Verification items for the finished model (mm, model axes). Round coordinates to 2 decimals unless told otherwise and drop trailing zeros. Order: outer loops, then holes, each group sorted by start corner. A loop starts at its lowest first (then second) coordinate and runs counter-clockwise, first axis right, second up. Notation, with made-up numbers: M 19,86.25 L 64,86.25 A28 ccw 64,122.25 Z; hole C 49,-30.5 d7. An arc over 180 degrees is marked long. Use one line per item in the form item = value. Start each with the question number.
Item 1: Thickness scan on probe 1 along Y at (x, z) = (-1.05, 21.75); probe 2 along X at (y, z) = (-1469, 3.25); probe 3 along Y at (x, z) = (1.15, 18.5). Record the ranges inside material, lowest first. Write a range as [from, to].
Item 2: Cross-section at B-B on y = -1652. Enter the section's corners in (x, z).
Item 3: Cross-section at A-A on z = 8.5. Enter the section's corners in (x, y), then the cut area to 3 significant figures.
Item 4: Go/stop test with a flat-tipped pin: pin 1 Ø2 at (x, y) = (-10, -1359.5) entering from -Z. Record where the tip stops, or that it passes through.
from build123d import *

# Parameters (mm, degrees)
F0_W     = 3.9
F0_H     = 3
F0_W_2   = 4.1
F0_H_2   = 5.1741511822
F1_DEPTH = 2000
F3_D     = 2
F4_W     = 32.8
F4_H     = 100
F5_DEPTH = 25.0010018114


with BuildPart() as f1:
    # F0 (on Front) → F1 (new body)
    with BuildSketch(Plane.XZ):
        with Locations((14.5, 1.7925839761)):
            Rectangle(F0_W, F0_H)
        Polygon((-16.35, 25.2925857875), (-16.35, 0.2925839761), (-12.45, 0.2925839761), (-12.45, 3.2925839761), (-12.45, 8.4667351583), (-8.35, 8.4667351583), (-8.35, 16.0925839761), (8.45, 16.0925839761), (8.45, 8.4667351583), (12.55, 8.4667351583), (12.55, 3.2925839761), (16.45, 3.2925839761), (16.45, 25.2925857875), align=None)
        with Locations((-10.4, 5.8796595672)):
            Rectangle(F0_W_2, F0_H_2)
        with Locations((10.5, 5.8796595672)):
            Rectangle(F0_W_2, F0_H_2)
    extrude(amount=F1_DEPTH)

    # F3 (through all)
    with Locations(Plane.XY.offset(25.2925857875)):
        with Locations((-1.05, -373), (1.15, -1627)):
            Hole(F3_D / 2)

    # F4 (on face) → F5 (cut, through all)
    with BuildSketch(Plane.XY.offset(25.2925857875)):
        with Locations((0.05, -50)):
            Rectangle(F4_W, F4_H)
        with Locations((0.05, -1950)):
            Rectangle(F4_W, F4_H)
    extrude(amount=-F5_DEPTH, mode=Mode.SUBTRACT)


solid = f1.part
Output values:
q1.probe_1 = [-1900, -374], [-372, -100]
q1.probe_2 = [-16.35, -12.45], [12.55, 16.45]
q1.probe_3 = [-1900, -1628], [-1626, -100]
q2.outline = M -16.35,0.29 L -12.45,0.29 L -12.45,3.29 L -8.35,3.29 L -8.35,16.09 L 8.45,16.09 L 8.45,3.29 L 12.55,3.29 L 12.55,0.29 L 16.45,0.29 L 16.45,25.29 L -16.35,25.29 Z
q3.outline = M -16.35,-1900 L -8.35,-1900 L -8.35,-100 L -16.35,-100 Z; M 8.45,-1900 L 16.45,-1900 L 16.45,-100 L 8.45,-100 Z
q3.area = 28,800 mm2
q4.pin_1 = 3.29
